Read the model definition and answer for the solid it produces. Units are mm, in the model's axes. Coordinates: 2 decimals unless noted, no trailing zeros. Write each loop counter-clockwise with the first axis right and the second up, starting at its lowest first coordinate (ties: lowest second). Pieces come first, ordered by that corner, then holes. Notation, with made-up numbers: (8.25, 51) -> (13.25, 51) arc R17 cw to (13.25, 75) -> close; hole circle Ø1 at (-9, -33). An arc over 180 degrees is marked (long way). One line per item, written item: value. Start each with the question number.
from build123d import *

# Parameters (mm, degrees)
SKETCH1_W               = 139.7
SKETCH1_H               = 42.8625
BOSS_EXTRUDE1_DEPTH     = 45.72
CUT_EXTRUDE2_DEPTH      = 40.64
CUT_EXTRUDE3_DEPTH      = 1
CUT_EXTRUDE3_DEPTH_BACK = 139.7


with BuildPart() as part:
    # Sketch1 → Boss-Extrude1 (new body)
    with BuildSketch(Plane(origin=(0, 0, 0), x_dir=(1, 0, 0), z_dir=(0, 1, 0))):
        with Locations((92.537965446, 28.29525747)):
            Rectangle(SKETCH1_W, SKETCH1_H)
    extrude(amount=BOSS_EXTRUDE1_DEPTH)

    # Sketch7 → Cut-Extrude2 (cut)
    with BuildSketch(Plane(origin=(0, 0, 0), x_dir=(1, 0, 0), z_dir=(0, 1, 0))):
        Polygon((22.687965446, 43.37650747), (29.037965446, 43.37650747), (29.037965446, 49.72650747), (156.037965446, 49.72650747), (156.037965446, 43.37650747), (162.387965446, 43.37650747), (162.387965446, 13.21400747), (156.037965446, 13.21400747), (156.037965446, 6.86400747), (29.037965446, 6.86400747), (29.037965446, 13.21400747), (22.687965446, 13.21400747), align=None)
    extrude(amount=CUT_EXTRUDE2_DEPTH, mode=Mode.SUBTRACT)

    # Sketch8 → Cut-Extrude3 (cut, two sides)
    with BuildSketch(Plane.ZY.offset(-22.687965446)) as cut_extrude3_sk:
        with BuildLine():
            Line((-13.21400747, 45.72), (-43.37650747, 45.72))
            add(Edge.make_bspline(
                [(-43.37650747, 45.72), (-28.29525747, 41.58097799), (-13.21400747, 45.72)],
                knots=[0, 0, 0, 1, 1, 1], degree=2))
        make_face()
    extrude(amount=CUT_EXTRUDE3_DEPTH, mode=Mode.SUBTRACT)
    extrude(cut_extrude3_sk.sketch, amount=-CUT_EXTRUDE3_DEPTH_BACK, mode=Mode.SUBTRACT)


solid = part.part
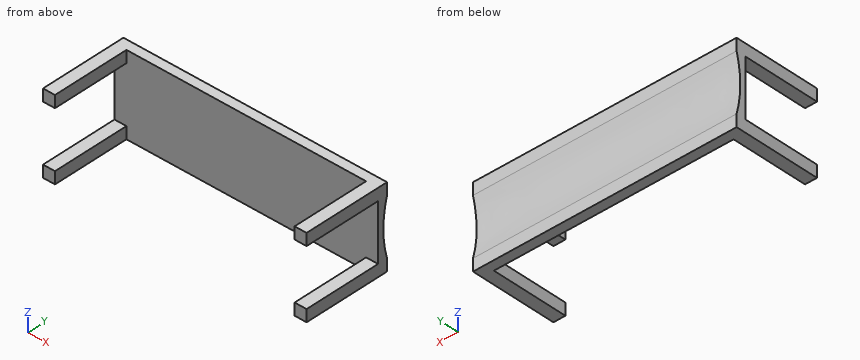
1. A cutting plane is placed at A-A on y = 21. Give the vertices of the cut face in (x, z).
2. Given pin 1 (10 mm diameter, centred on y = 8.5, z = -35.5, fed in from -X); pin 2 (13 mm diameter, centred on x = 95, z = -31.5, fed in from -Y); pin 3 (12 mm diameter, centred on x = 37.5, z = -31.5, fed in from +Y), each flat-ended and moving along its own axis, determine where each tip first touches the part or whether it passes through.
3. A cutting plane is placed at B-B on z = -11.5. Give the vertices of the cut face in (x, y).
4. Find the intervals of material crossed by probe 1 along X at (y, z) = (7.5, -45); probe 2 along Y at (x, z) = (34, -47); probe 3 along Y at (x, z) = (65, -23.5), in increasing order. Write a range as from..to.
Derived:
1. outline: (22.69, -49.73) -> (29.04, -49.73) -> (29.04, -43.38) -> (22.69, -43.38) -> close; (22.69, -13.21) -> (29.04, -13.21) -> (29.04, -6.86) -> (22.69, -6.86) -> close; (156.04, -49.73) -> (162.39, -49.73) -> (162.39, -43.38) -> (156.04, -43.38) -> close; (156.04, -13.21) -> (162.39, -13.21) -> (162.39, -6.86) -> (156.04, -6.86) -> close
2. pin 1: passes through
2. pin 2: stops at y = 40.64
2. pin 3: stops at y = 44.42
3. outline: (22.69, 0) -> (29.04, 0) -> (29.04, 40.64) -> (156.04, 40.64) -> (156.04, 0) -> (162.39, 0) -> (162.39, 45.72) -> (22.69, 45.72) -> close
4. probe 1: x = 22.69..29.04, 156.04..162.39
4. probe 2: y = 40.64..45.72
4. probe 3: y = 40.64..43.86
